```python
from build123d import *

# Parameters (mm, degrees)
SKETCH_1_W          = 59.5
SKETCH_1_H          = 19
SKETCH_1_R          = 1.5
EXTRUDE_1_DEPTH     = 4
SKETCH_2_W          = 4
SKETCH_2_H          = 19
EXTRUDE_2_DEPTH     = 24
SKETCH_3_W          = 3
SKETCH_3_H          = 19
EXTRUDE_3_DEPTH     = 48
SKETCH_4_R          = 2.5
CUT_EXTRUDE_1_DEPTH = 48
SKETCH_5_R          = 1.5
CUT_EXTRUDE_2_DEPTH = 48
CHAMFER_1_SIZE      = 2
FILLET_1_R          = 1


with BuildPart() as part:
    # 草图1 → 凸台-拉伸1 (new body)
    with BuildSketch(Plane.XY):
        with Locations((10.493245584, -4.144948765)):
            Rectangle(SKETCH_1_W, SKETCH_1_H)
        with Locations((-10.256754416, 1.355051235)):
            Circle(SKETCH_1_R, mode=Mode.SUBTRACT)
        with Locations((26.243245584, 1.355051235)):
            Circle(SKETCH_1_R, mode=Mode.SUBTRACT)
    extrude(amount=EXTRUDE_1_DEPTH)

    # 草图2 → 凸台-拉伸2 (add)
    with BuildSketch(Plane.XY.offset(4)):
        with Locations((-17.256754416, -4.144948765)):
            Rectangle(SKETCH_2_W, SKETCH_2_H)
    extrude(amount=EXTRUDE_2_DEPTH)

    # 草图3 → 凸台-拉伸3 (add)
    with BuildSketch(Plane.XY.offset(4)):
        with Locations((38.743245584, -4.144948765)):
            Rectangle(SKETCH_3_W, SKETCH_3_H)
    extrude(amount=EXTRUDE_3_DEPTH)

    # 草图4 → 切除-拉伸1 (cut)
    with BuildSketch(Plane(origin=(-15.256754416, 0, 0), x_dir=(0, 0, -1), z_dir=(1, 0, 0))):
        with Locations((-22, -3.644948765)):
            Circle(SKETCH_4_R)
    extrude(amount=-CUT_EXTRUDE_1_DEPTH, mode=Mode.SUBTRACT)

    # 草图5 → 切除-拉伸2 (cut)
    with BuildSketch(Plane.ZY.offset(-37.243245584)):
        with Locations((11, -3.644948765)):
            Circle(SKETCH_5_R)
        with Locations((47.5, -3.644948765)):
            Circle(SKETCH_5_R)
    extrude(amount=-CUT_EXTRUDE_2_DEPTH, mode=Mode.SUBTRACT)

    # 倒角1
    chamfer_1_edges = [part.edges().sort_by_distance(p)[0] for p in [
        (-15.256754416, -4.144948765, 4),
        (37.243245584, -4.144948765, 4),
        (-19.256754416, -4.144948765, 0),
        (40.243245584, -4.144948765, 0),
    ]]
    chamfer(chamfer_1_edges, length=CHAMFER_1_SIZE)

    # 圆角1
    fillet_1_edges = [part.edges().sort_by_distance(p)[0] for p in [
        (-17.256754416, -13.644948765, 28),
        (-15.256754416, -4.144948765, 28),
        (-15.256754416, -13.644948765, 17),
        (-19.256754416, -4.144948765, 28),
        (37.243245584, -13.644948765, 29),
        (37.243245584, -4.144948765, 52),
        (38.743245584, -13.644948765, 52),
        (40.243245584, -4.144948765, 52),
        (40.243245584, -4.144948765, 2),
        (10.493245584, -13.644948765, 0),
        (-17.256754416, -4.144948765, 0),
        (38.243245584, -4.144948765, 0),
        (10.993245584, -13.644948765, 4),
        (-18.256754416, -13.644948765, 1),
        (39.243245584, -13.644948765, 1),
        (-19.256754416, -4.144948765, 2),
        (37.243245584, -4.144948765, 6),
        (-13.256754416, -4.144948765, 4),
        (35.243245584, -4.144948765, 4),
        (-15.256754416, -4.144948765, 6),
        (40.243245584, -13.644948765, 27),
        (36.243245584, -13.644948765, 5),
        (-19.256754416, -13.644948765, 15),
        (-14.256754416, -13.644948765, 5),
    ]]
    fillet(fillet_1_edges, radius=FILLET_1_R)


solid = part.part
```
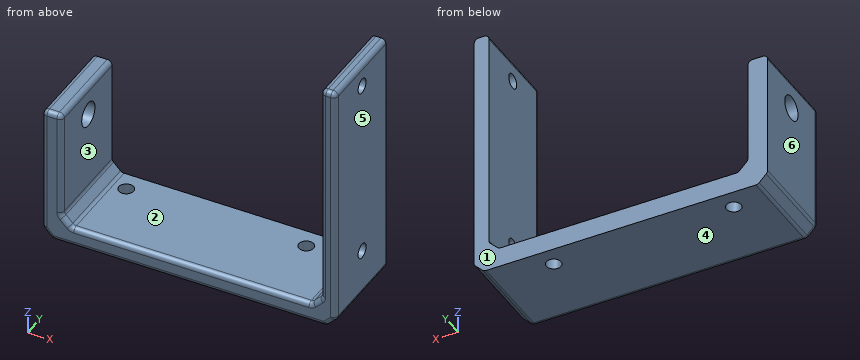
For this review, take the finished solid that the model builds, in its own axes (mm). Face numbers are marked on the shaded views. A direction names the side the tool comes from. Coordinates: 2 decimals unless noted, no trailing zeros. Loops run counter-clockwise (first coordinate to the right, second up) from the corner with the lowest first, then second, coordinate; pieces in that order, holes last. Notation, with made-up numbers: (-2.5, 80.25) -> (44.5, 80.25) arc R18 ccw to (44.5, 115.25) -> close; hole circle Ø11 at (75.5, 51.25). An arc over 180 degrees is marked (long way). Return JSON: item names as keys, results as strings. Group by question number.
(1) Consider section C-C, the plane x = -0.5. Give the boundary of the cut face in (y, z), plus the area to 3 significant figures.
(2) Mouldability with a two-part tool opening along X and no side actions: class the marked faces 3, 4, 5 and 6 as pulls with the +X half, pulls with the -X half, needs draft (parallel to the pull), parting line crosses it, or undercut.
(3) Consider section B-B, the plane z = 8. Give the boundary of the cut face in (x, y).
(4) Consider section A-A, the plane z = 22. Give the boundary of the cut face in (x, y).
(5) To check wall thickness, follow L1, parallel to Y at x = 39.35, z = 47.5; L2, parallel to X at y = -10.25, z = 15.5; L3, parallel to Z at x = -17, y = 1.75. State the ranges of each line that lie inside material, in increasing order.
(6) Consider section D-D, the plane y = -8.5. Give the boundary of the cut face in (x, z).
(7) Tool access review of the marked faces 1 and 2: name each direction out of +Z, -Z, +X, -X, +Y, -Y from which nothing blocks a thin tool from reaching the whole face with its end or side.
(8) For pin 1 Ø2 at (x, y) = (2.5, -1.5) entering from +Z; pin 2 Ø1.5 at (y, z) = (2.5, 41) entering from -X; pin 3 Ø0.6 at (x, y) = (-17.5, -3) entering from +Z; pin 4 Ø6 at (y, z) = (-3.64, 22) entering from -X, all flat-tipped, find the tip position at first contact; note any pin that passes through.
Results below:
{
 "1": {"outline": "(-13.64, 1) arc R1 ccw to (-12.64, 0) -> (5.36, 0) -> (5.36, 4) -> (-12.64, 4) arc R1 ccw to (-13.64, 3) -> close", "area": "75.6 mm2"},
 "2": {"face 3": "undercut", "face 4": "needs draft", "face 5": "pulls with the +X half", "face 6": "pulls with the -X half"},
 "3": {"outline": "(-19.26, -12.64) arc R1 ccw to (-18.26, -13.64) -> (-16.26, -13.64) arc R1 ccw to (-15.26, -12.64) -> (-15.26, 5.36) -> (-19.26, 5.36) -> close; (37.24, -12.64) arc R1 ccw to (38.24, -13.64) -> (39.24, -13.64) arc R1 ccw to (40.24, -12.64) -> (40.24, 5.36) -> (37.24, 5.36) -> close"},
 "4": {"outline": "(-19.26, -12.64) arc R1 ccw to (-18.26, -13.64) -> (-16.26, -13.64) arc R1 ccw to (-15.26, -12.64) -> (-15.26, -6.14) -> (-19.26, -6.14) -> close; (-19.26, -1.14) -> (-15.26, -1.14) -> (-15.26, 5.36) -> (-19.26, 5.36) -> close; (37.24, -12.64) arc R1 ccw to (38.24, -13.64) -> (39.24, -13.64) arc R1 ccw to (40.24, -12.64) -> (40.24, 5.36) -> (37.24, 5.36) -> close"},
 "5": {"L1": "y = -13.64 to -5.14, -2.14 to 5.36", "L2": "x = -19.26 to -15.26, 37.24 to 40.24", "L3": "z = 0.01 to 28"},
 "6": {"outline": "(-19.26, 2.41) arc R1 ccw to (-18.96, 1.71) -> (-17.55, 0.29) arc R1 ccw to (-16.84, 0) -> (37.83, 0) arc R1 ccw to (38.54, 0.29) -> (39.95, 1.71) arc R1 ccw to (40.24, 2.41) -> (40.24, 51) arc R1 ccw to (39.24, 52) -> (38.24, 52) arc R1 ccw to (37.24, 51) -> (37.24, 6.41) arc R1 cw to (36.95, 5.71) -> (35.54, 4.29) arc R1 cw to (34.83, 4) -> (-12.84, 4) arc R1 cw to (-13.55, 4.29) -> (-14.96, 5.71) arc R1 cw to (-15.26, 6.41) -> (-15.26, 27) arc R1 ccw to (-16.26, 28) -> (-18.26, 28) arc R1 ccw to (-19.26, 27) -> close"},
 "7": {"face 1": "+Z, -Z, +X, -X, +Y", "face 2": "+Z, +Y, -Y"},
 "8": {"pin 1": "stops at z = 4", "pin 2": "stops at x = 37.24", "pin 3": "stops at z = 28", "pin 4": "stops at x = -19.26"}
}
